from build123d import *

# Parameters (mm, degrees)
SKETCH1_R           = 100
SKETCH1_R_2         = 2
SKETCH1_W           = 6.5
SKETCH1_H           = 12.5
BOSS_EXTRUDE1_DEPTH = 5
SKETCH1_3_R         = 2
BOSS_EXTRUDE2_DEPTH = 4
SKETCH1_4_R         = 2
BOSS_EXTRUDE3_DEPTH = 1
SKETCH1_6_R         = 2
BOSS_EXTRUDE6_DEPTH = 5
SKETCH1_7_R         = 2
CUT_EXTRUDE1_DEPTH  = 3


with BuildPart() as part:
    # Sketch1 → Boss-Extrude1 (new body)
    with BuildSketch(Plane.XY):
        Circle(SKETCH1_R)
        with BuildLine():
            Line((-17.3, 3.6), (-14.149204925, 3.6))
            ThreePointArc((-14.149204925, 3.6), (0, 14.6), (14.149204925, 3.6))
            Line((14.149204925, 3.6), (17.3, 3.6))
            ThreePointArc((17.3, 3.6), (20.9, 0), (17.3, -3.6))
            Line((17.3, -3.6), (14.149204925, -3.6))
            ThreePointArc((14.149204925, -3.6), (12.316145556, -7.840443778), (9.25, -11.295906338))
            Line((9.25, -11.295906338), (9.25, -15.647016094))
            Line((9.25, -15.647016094), (8.1, -15.647016094))
            Line((8.1, -15.647016094), (8.1, -30.2))
            Line((8.1, -30.2), (-8.1, -30.2))
            Line((-8.1, -30.2), (-8.1, -15.647016094))
            Line((-8.1, -15.647016094), (-9.25, -15.647016094))
            Line((-9.25, -15.647016094), (-9.25, -11.295906338))
            ThreePointArc((-9.25, -11.295906338), (-12.316145556, -7.840443778), (-14.149204925, -3.6))
            Line((-14.149204925, -3.6), (-17.3, -3.6))
            ThreePointArc((-17.3, -3.6), (-20.9, 0), (-17.3, 3.6))
        make_face(mode=Mode.SUBTRACT)
        with Locations((0, 32)):
            Circle(SKETCH1_R_2, mode=Mode.SUBTRACT)
        with Locations((0, 44)):
            Rectangle(SKETCH1_W, SKETCH1_H, mode=Mode.SUBTRACT)
        with Locations((0, 56)):
            Circle(SKETCH1_R_2, mode=Mode.SUBTRACT)
    extrude(amount=BOSS_EXTRUDE1_DEPTH)

    # Sketch1<3> → Boss-Extrude2 (add)
    # profile 1 of 2: a face of its own
    with BuildSketch(Plane.XY):
        with BuildLine():
            ThreePointArc((-14.149204925, -3.6), (-14.6, 0), (-14.149204925, 3.6))
            Line((-14.149204925, 3.6), (-17.3, 3.6))
            ThreePointArc((-17.3, 3.6), (-20.9, 0), (-17.3, -3.6))
            Line((-17.3, -3.6), (-14.149204925, -3.6))
        make_face()
        with Locations((-17.5, 0)):
            Circle(SKETCH1_3_R, mode=Mode.SUBTRACT)
    # profile 2 of 2: a face of its own
    with BuildSketch(Plane.XY):
        with BuildLine():
            Line((17.3, 3.6), (14.149204925, 3.6))
            ThreePointArc((14.149204925, 3.6), (14.6, 0), (14.149204925, -3.6))
            Line((14.149204925, -3.6), (17.3, -3.6))
            ThreePointArc((17.3, -3.6), (20.9, 0), (17.3, 3.6))
        make_face()
        with Locations((17.5, 0)):
            Circle(SKETCH1_3_R, mode=Mode.SUBTRACT)
    extrude(amount=BOSS_EXTRUDE2_DEPTH)

    # Sketch1<4> → Boss-Extrude3 (add)
    with BuildSketch(Plane.XY):
        with Locations((-17.5, 0)):
            Circle(SKETCH1_4_R)
        with Locations((17.5, 0)):
            Circle(SKETCH1_4_R)
    extrude(amount=BOSS_EXTRUDE3_DEPTH)

    # Sketch1<6> → Boss-Extrude6 (add)
    with BuildSketch(Plane.XY):
        with Locations((0, 56)):
            Circle(SKETCH1_6_R)
        with Locations((0, 32)):
            Circle(SKETCH1_6_R)
    extrude(amount=BOSS_EXTRUDE6_DEPTH)

    # Sketch1<7> → Cut-Extrude1 (cut)
    with BuildSketch(Plane.XY):
        with Locations((0, 32)):
            Circle(SKETCH1_7_R)
        with Locations((0, 56)):
            Circle(SKETCH1_7_R)
    extrude(amount=CUT_EXTRUDE1_DEPTH, mode=Mode.SUBTRACT)


solid = part.part
For this review, take the finished solid that the model builds, in its own axes (mm). A direction names the side the tool comes from. Coordinates: 2 decimals unless noted, no trailing zeros. Order: outer loops, then holes, each group sorted by start corner. A loop starts at its lowest first (then second) coordinate and runs counter-clockwise, first axis right, second up. Notation, with made-up numbers: (19, 26.5) - (39, 26.5) arc R14 cw to (39, 41.5) - close; hole circle Ø10 at (-19, 87). An arc over 180 degrees is marked (long way). Answer as CSV lines item,"result". Start each with the question number.
1) Machinability: for faces 5 (the flat face through (-15, 0, 4)), 6 (the flat face through (8.1, -23, 2)), 7 (the flat face through (21, 1, 5)), which of the approach directions +Z, -Z, +X, -X, +Y, -Y give a long, thin tool a straight path to every point of the face, cutting with its end or side? Answer none if there is none.
2) Add section B-B (x = -50). State the section outline as (y, z) points, then the cut area to 3 significant figures.
3) Add section A-A (z = 1.9). State the section outline as (x, y) points, then the cut area to 3 significant figures.
4) Draft analysis for pull direction X (two halves, no side actions). For faces 1 (the flat face through (21, 1, 0)), 2 (the flat face through (-3.25, 44, 2)), 3 (the flat face through (0, 50.25, 2)), 4 (the cylindrical face through (95.38, 30.04, 2.46)), state which applies: +X half, -X half, draft (parallel to the pull), parting line (faces both ways), or undercut.
5) To check wall thickness, follow line 1 along Y through (x, z) = (0, 2.2); line 2 along X through (y, z) = (-29.5, 4.45); line 3 along Y through (x, z) = (13, 4.5). State the ranges of each line that lie inside material, in increasing order. Write a range as [from, to].
6) Insertion check: P1, Ø7.5, axis at x = 16, y = 0, coming from the +Z side; P2, Ø2, axis at y = -22.5, z = 3.5, coming from the -X side; P3, Ø3, axis at y = -43.5, z = 1.5, coming from the -X side; P4, Ø2, axis at y = -14, z = 1.5, coming from the +X side. Each pin has a flat end and moves straight along its axis. Give the tip position at first contact, or say it passes through.
7) Add section C-C (y = -35.5). State the section outline as (x, z) points.
Result:
1,face 5,"+Z"
1,face 6,"+Z, -Z"
1,face 7,"+Z, +X, -X, +Y, -Y"
2,outline,"(-86.6, 0) - (86.6, 0) - (86.6, 5) - (-86.6, 5) - close"
2,area,"866 mm^2"
3,outline,"circle Ø200 at (0, 0); hole circle Ø4 at (-17.5, 0); hole (-9.25, -15.65) - (-8.1, -15.65) - (-8.1, -30.2) - (8.1, -30.2) - (8.1, -15.65) - (9.25, -15.65) - (9.25, -11.3) arc R14.6 ccw (long way) to (-9.25, -11.3) - close; hole (-3.25, 37.75) - (3.25, 37.75) - (3.25, 50.25) - (-3.25, 50.25) - close; hole circle Ø4 at (0, 32); hole circle Ø4 at (0, 56); hole circle Ø4 at (17.5, 0)"
3,area,"30,300 mm^2"
4,face 1,"draft"
4,face 2,"undercut"
4,face 3,"undercut"
4,face 4,"parting line"
5,line 1,"[-100, -30.2], [14.6, 30], [34, 37.75], [50.25, 54], [58, 100]"
5,line 2,"[-95.55, -8.1], [8.1, 95.55]"
5,line 3,"[-99.15, -6.65], [6.65, 99.15]"
6,P1,"z = 5"
6,P2,"x = -97.66"
6,P3,"x = -90.75"
6,P4,"x = 99.15"
7,outline,"(-93.49, 0) - (93.49, 0) - (93.49, 5) - (-93.49, 5) - close"
